CAD build for the part. Positions are in the model's coordinates, mm. Face numbers are marked on the shaded views. A direction names the side the tool comes from. Round coordinates to 2 decimals unless told otherwise and drop trailing zeros. Order: outer loops, then holes, each group sorted by start corner. A loop starts at its lowest first (then second) coordinate and runs counter-clockwise, first axis right, second up. Notation, with made-up numbers: M 16,10.25 L 48,10.25 A20 cw 48,27.25 Z; hole C -3.75,62.5 d10. An arc over 180 degrees is marked long. Put each result on its own line as item: value.
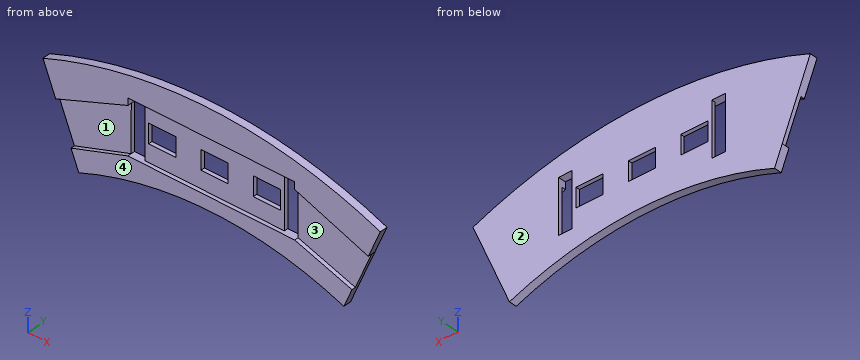
```python
from build123d import *

# Parameters (mm, degrees)
F1_DEPTH = 2
F0_W     = 36
F0_H     = 14
F0_W_2   = 7
F0_H_2   = 5
F2_DEPTH = 1
F3_DEPTH = 2
F4_DEPTH = 1
F5_DEPTH = 1
F6_DEPTH = 2.001
F7_DEPTH = 2.001
F8_DEPTH = 1


# Not quite as in the source:
# - ends of sketch curves that miss each other by under 0.0002 mm in the source are joined


with BuildPart() as f1:
    # F0 (on Front) → F1 (new body)
    with BuildSketch(Plane.XZ):
        with BuildLine():
            Line((40.4628534786, 0), (43.5572046873, 7.3690142199))
            ThreePointArc((43.5572046873, 7.3690142199), (0.1833509298, 16.332060188), (-43.3610966095, 8.2383298181))
            Line((-43.3610966095, 8.2383298181), (-40.0939611875, 0))
            Line((-40.0939611875, 0), (-21.4795553588, 7.1586821743))
            Line((-21.4795553588, 7.1586821743), (-21.4764592054, 9.000000095))
            Line((-21.4764592054, 9.000000095), (-18, 9.000000095))
            Line((-18, 9.000000095), (18, 9.000000095))
            Line((18, 9.000000095), (21.5, 9.000000095))
            Line((21.5, 9.000000095), (21.5, 7.1586821743))
            Line((21.5, 7.1586821743), (40.4628534786, 0))
        make_face()
    extrude(amount=F1_DEPTH)

    # F0 (on Front) → F2 (join)
    with BuildSketch(Plane.XZ):
        Polygon((21.5, -4.999999905), (21.5, 7.1586821743), (21.5, 9.000000095), (18, 9.000000095), (18, -4.999999905), align=None)
        with Locations((0, 2.000000095)):
            Rectangle(F0_W, F0_H)
        with Locations((-13.5, 2.000000095)):
            Rectangle(F0_W_2, F0_H_2, mode=Mode.SUBTRACT)
        with Locations((0, 2.000000095)):
            Rectangle(F0_W_2, F0_H_2, mode=Mode.SUBTRACT)
        Polygon((17, 4.500000095), (17, -0.499999905), (15, -0.499999905), (10, -0.499999905), (10, 2.500000095), (10, 4.500000095), align=None, mode=Mode.SUBTRACT)
        Polygon((-21.4764592054, 9.000000095), (-21.4795553588, 7.1586821743), (-21.5, -4.9999801132), (-18, -4.999999905), (-18, 9.000000095), align=None)
    extrude(amount=F2_DEPTH)

    # F0 (on Front) → F3 (join)
    with BuildSketch(Plane.XZ):
        with BuildLine():
            Line((34.164145572, -15), (36.2637148742, -10))
            Line((36.2637148742, -10), (21.5, -4.999999905))
            Line((21.5, -4.999999905), (18, -4.999999905))
            Line((18, -4.999999905), (-18, -4.999999905))
            Line((-18, -4.999999905), (-21.5, -4.999999905))
            Line((-21.5, -4.999999905), (-36.1281871846, -10))
            Line((-36.1281871846, -10), (-34.1453001831, -15))
            ThreePointArc((-34.1453001831, -15), (0.0094226944, -8.3568901314), (34.164145572, -15))
        make_face()
    extrude(amount=F3_DEPTH)

    # F0 (on Front) → F4 (join)
    with BuildSketch(Plane.XZ):
        Polygon((36.2637148742, -10), (40.4628534786, 0), (21.5, 7.1586821743), (21.5, -4.999999905), align=None)
    extrude(amount=F4_DEPTH)

    # F0 (on Front) → F5 (join)
    with BuildSketch(Plane.XZ):
        Polygon((-21.4795553588, 7.1586821743), (-40.0939611875, 0), (-36.1281871846, -10), (-21.5, -4.999999905), align=None)
    extrude(amount=F5_DEPTH)

    # F0 (on Front) → F6 (cut, through all)
    with BuildSketch(Plane.XZ):
        Polygon((21.5, -4.999999905), (21.5, 7.1586821743), (21.5, 9.000000095), (18, 9.000000095), (18, -4.999999905), align=None)
    extrude(amount=F6_DEPTH, mode=Mode.SUBTRACT)

    # F0 (on Front) → F7 (cut, through all)
    with BuildSketch(Plane.XZ):
        Polygon((-21.4764592054, 9.000000095), (-21.4795553588, 7.1586821743), (-21.5, -4.9999801132), (-18, -4.999999905), (-18, 9.000000095), align=None)
    extrude(amount=F7_DEPTH, mode=Mode.SUBTRACT)

    # F0 (on Front) → F8 (join)
    with BuildSketch(Plane.XZ):
        with Locations((0, 2.000000095)):
            Rectangle(F0_W, F0_H)
        with Locations((-13.5, 2.000000095)):
            Rectangle(F0_W_2, F0_H_2, mode=Mode.SUBTRACT)
        with Locations((0, 2.000000095)):
            Rectangle(F0_W_2, F0_H_2, mode=Mode.SUBTRACT)
        Polygon((17, 4.500000095), (17, -0.499999905), (15, -0.499999905), (10, -0.499999905), (10, 2.500000095), (10, 4.500000095), align=None, mode=Mode.SUBTRACT)
    extrude(amount=F8_DEPTH)


solid = f1.part
```
Item 1: Tool access for the marked faces 1 and 2: list every direction of +Z, -Z, +X, -X, +Y, -Y with a clear straight run to the whole face (end or side of a thin tool).
Answers below:
face 1: -Y
face 2: +Z, -Z, +X, -X, +Y
Item 2: Probe line 1 along X through (y, z) = (-0.25, -4); line 2 along X through (y, z) = (-0.05, 1); line 3 along Z through (x, y) = (-15, -0.4). List the from-to ranges inside material, lowest first. Write a range as [from, to].
Answers below:
line 1: [-38.51, -21.5], [-18, 18], [21.5, 38.78]
line 2: [-40.49, -21.49], [-18, -17], [-10, -3.5], [3.5, 10], [17, 18], [21.5, 40.88]
line 3: [-9.6, -0.5], [4.5, 15.48]
Item 3: Mould opens along X. For the marked faces 3 and 4 say: pulls with the +X half, pulls with the -X half, needs draft (parallel to the pull), parting line crosses it, or undercut.
Answers below:
face 3: undercut
face 4: needs draft
Item 4: Band-saw the part on D-D on z = -6. Give the cut face in (x, y), and give its area (3 significant figures).
Answers below:
outline: M -37.71,-1 L -24.43,-1 L -24.43,-2 L 24.45,-2 L 24.45,-1 L 37.94,-1 L 37.94,0 L -37.71,0 Z
area: 125 mm²
Item 5: Pin check, flat tips, straight feed: P1, Ø6, axis at x = -25, z = 11, coming from the +Y side; P2, Ø0.8, axis at y = -0.5, z = 1.5, coming from the +X side; P3, Ø1.1, axis at x = -1, y = -0.5, coming from the +Z side; P4, Ø0.8, axis at x = -15, y = -0.5, coming from the +Z side. Stop position of each tip, or through.
Answers below:
P1: y = 0
P2: x = 41.26
P3: z = 16.34
P4: z = 15.53
Item 6: Band-saw the part on A-A on y = -1.55. Give the cut face in (x, z).
Answers below:
outline: M -43.36,8.24 L -40.09,0 L -21.48,7.16 L -21.48,9 L 21.5,9 L 21.5,7.16 L 40.46,0 L 43.56,7.37 A115 ccw Z; M -36.13,-10 L -34.15,-15 A91.12 cw 34.16,-15 L 36.26,-10 L 21.5,-5 L -21.5,-5 Z
Item 7: Band-saw the part on B-B on z = -1.5. Give the cut face in (x, y), and give its area (3 significant figures).
Answers below:
outline: M -39.5,-1 L -21.49,-1 L -21.49,0 L -39.5,0 Z; M -18,-1 L 18,-1 L 18,0 L -18,0 Z; M 21.5,-1 L 39.83,-1 L 39.83,0 L 21.5,0 Z
area: 72.3 mm²
Item 8: Band-saw the part on C-C on x = 25. Give the cut face in (y, z), and give its area (3 significant figures).
Answers below:
outline: M -2,-11.85 L 0,-11.85 L 0,13.37 L -2,13.37 L -2,5.84 L -1,5.84 L -1,-6.19 L -2,-6.19 Z
area: 38.4 mm²
